from build123d import *

# Parameters (mm, degrees)
CYLINDER011_R     = 1
CYLINDER011_DEPTH = 10
CYLINDER012_R     = 1
CYLINDER012_DEPTH = 10
BOX014_W          = 5
BOX014_H          = 5
BOX014_DEPTH      = 5
FILLET005_R       = 2
BOX013_W          = 5
BOX013_H          = 5
BOX013_DEPTH      = 5
FILLET004_R       = 2
BOX016_W          = 64
BOX016_H          = 2
BOX016_DEPTH      = 115


with BuildPart() as cilindro011:
    # Cylinder011 → Cylinder011 (new body)
    with BuildSketch(Plane(origin=(59, 6, 106), x_dir=(0, 0, 1), z_dir=(0, 1, 0))):
        Circle(CYLINDER011_R)
    extrude(amount=CYLINDER011_DEPTH)


with BuildPart() as cilindro012:
    # Cylinder012 → Cylinder012 (new body)
    with BuildSketch(Plane(origin=(55, 6, 106), x_dir=(0, 0, 1), z_dir=(0, 1, 0))):
        Circle(CYLINDER012_R)
    extrude(amount=CYLINDER012_DEPTH)


with BuildPart() as fillet005:
    # Box014 → Box014 (new body)
    with BuildSketch(Plane(origin=(57, 6, 108), x_dir=(1, 0, 0), z_dir=(0, 0, 1))):
        with Locations((2.5, 2.5)):
            Rectangle(BOX014_W, BOX014_H)
    extrude(amount=BOX014_DEPTH)

    # Fillet005
    fillet005_edges = [fillet005.edges().sort_by_distance(p)[0] for p in [
        (57, 8.5, 113),
        (57, 8.5, 108),
        (62, 8.5, 113),
        (62, 8.5, 108),
    ]]
    fillet(fillet005_edges, radius=FILLET005_R)


with BuildPart() as fillet005_1:
    # Fillet005 placement: moved
    add(fillet005.part.moved(Location((-8, 0, 0))))


with BuildPart() as fillet004:
    # Box013 → Box013 (new body)
    with BuildSketch(Plane(origin=(57, 6, 108), x_dir=(1, 0, 0), z_dir=(0, 0, 1))):
        with Locations((2.5, 2.5)):
            Rectangle(BOX013_W, BOX013_H)
    extrude(amount=BOX013_DEPTH)

    # Fillet004
    fillet004_edges = [fillet004.edges().sort_by_distance(p)[0] for p in [
        (57, 8.5, 113),
        (57, 8.5, 108),
        (62, 8.5, 113),
        (62, 8.5, 108),
    ]]
    fillet(fillet004_edges, radius=FILLET004_R)


with BuildPart() as back:
    # Box016 → Box016 (new body)
    with BuildSketch(Plane(origin=(0, 7, 0), x_dir=(1, 0, 0), z_dir=(0, 0, 1))):
        with Locations((32, 1)):
            Rectangle(BOX016_W, BOX016_H)
    extrude(amount=BOX016_DEPTH)

    # Cut020: cut Fillet004
    add(fillet004.part, mode=Mode.SUBTRACT)

    # Cut021: cut Fillet005
    add(fillet005_1.part, mode=Mode.SUBTRACT)

    # Cut031: cut Cilindro012
    add(cilindro012.part, mode=Mode.SUBTRACT)

    # Cut032: cut Cilindro011
    add(cilindro011.part, mode=Mode.SUBTRACT)


solid = back.part
The listing builds one solid part. Answer for the finished solid, in the listing's coordinates (mm). A direction names the side the tool comes from. Coordinates: 2 decimals unless noted, no trailing zeros. Answer in a Markdown table with one row per item.
1) Which of the six approach directions +Z, -Z, +X, -X, +Y, -Y give full straight-line access (tool end or side, diameter ignored) to faces 5 (the flat face through (32, 7, 57)), 6 (the cylindrical face through (61.43, 8.01, 112.4))?
Answers below:
| item | result |
|---|---|
| face 5 | +Z, -Z, +X, -X, -Y |
| face 6 | +Y, -Y |
2) Find the intervals of material crossed by probe 1 along X at (y, z) = (7.9, 106); probe 2 along Z at (x, y) = (59, 7.7); probe 3 along Z at (x, y) = (55, 8.2), in increasing order.
Answers below:
| item | result |
|---|---|
| probe 1 | 0 to 54, 56 to 58, 60 to 64 |
| probe 2 | 0 to 105, 107 to 108, 113 to 115 |
| probe 3 | 0 to 105, 107 to 115 |
3) Determine the mould class of faces 1 (the flat face through (32, 8, 115)), 2 (the flat face through (0, 8, 57)), 3 (the flat face through (64, 8, 57)), 4 (the cylindrical face through (49.57, 8.01, 112.4)) for opening direction X: released by +X, released by -X, zero draft, split by the parting line, or undercut.
Answers below:
| item | result |
|---|---|
| face 1 | zero draft |
| face 2 | released by -X |
| face 3 | released by +X |
| face 4 | undercut |
4) Given pin 1 (0.8 mm diameter, centred on x = 59.5, y = 8, fed in from -Z); pin 2 (1.2 mm diameter, centred on x = 59, z = 106, fed in from -Y) (3 decimals), each flat-ended and moving along its own axis, determine where each tip first touches the part or whether it passes through.
Answers below:
| item | result |
|---|---|
| pin 1 | z = 0 |
| pin 2 | through |
